Could you check a few things on this model? Use its own coordinates, in mm. A direction names the side the tool comes from. Round coordinates to 2 decimals unless told otherwise and drop trailing zeros. Answer in a Markdown table with one row per item.
Autodesk Fusion 360 part; units mm, degrees
sketch "Sketch1" plane through (0, 0, 0) normal (0, 1, 0) x (1, 0, 0)
  spline S0 degree 3 poles (0, -3.15) (-1.7568, -3.15) (-3.175, -1.7318) (-3.175, 0.025) knots 0 0 0 0 1 1 1 1
  spline S1 degree 3 poles (-3.175, 0.025) (-3.175, 1.7818) (-1.7568, 3.2) (0, 3.2) knots 0 0 0 0 1 1 1 1
  spline S2 degree 3 poles (0, 3.2) (1.7568, 3.2) (3.175, 1.7818) (3.175, 0.025) knots 0 0 0 0 1 1 1 1
  spline S3 degree 3 poles (3.175, 0.025) (3.175, -1.7318) (1.7568, -3.15) (0, -3.15) knots 0 0 0 0 1 1 1 1
  spline S4 degree 3 poles (0, -2.7769) (0.3175, -2.7769) (0.6244, -2.7187) (0.9075, -2.6208) knots 0 0 0 0 1 1 1 1
  line L0 (0.9075, -2.6208) -> (0.0344, -0.7344)
  spline S5 degree 3 poles (0.0344, -0.7344) (0.0238, -0.7238) (0.0238, -0.7) (0, -0.7) knots 0 0 0 0 1 1 1 1
  spline S6 degree 3 poles (0, -0.7) (-0.0238, -0.7) (-0.0238, -0.7238) (-0.0344, -0.7344) knots 0 0 0 0 1 1 1 1
  line L1 (-0.0344, -0.7344) -> (-0.9075, -2.6208)
  line L2 (-1.3494, -2.425) -> (-0.3387, -0.2475)
  spline S7 degree 3 poles (-0.3387, -0.2475) (-0.3175, -0.2025) (-0.2937, -0.1893) (-0.2646, -0.1893) knots 0 0 0 0 1 1 1 1
  line L3 (-0.2646, -0.1893) -> (0.2646, -0.1893)
  spline S8 degree 3 poles (0.2646, -0.1893) (0.2963, -0.1893) (0.3175, -0.2025) (0.3413, -0.2475) knots 0 0 0 0 1 1 1 1
  line L4 (0.3413, -0.2475) -> (1.3388, -2.425)
  spline S9 degree 3 poles (1.3388, -2.425) (1.7568, -2.1869) (2.1167, -1.8456) (2.3707, -1.4381) knots 0 0 0 0 1 1 1 1
  line L5 (2.3707, -1.4381) -> (0.9525, 1.3056)
  spline S10 degree 3 poles (0.9525, 1.3056) (0.9419, 1.3294) (0.926, 1.34) (0.9181, 1.34) knots 0 0 0 0 1 1 1 1
  spline S11 degree 3 poles (0.9181, 1.34) (0.8969, 1.34) (0.8969, 1.3188) (0.8837, 1.3056) knots 0 0 0 0 1 1 1 1
  line L6 (0.8837, 1.3056) -> (0.3413, 0.1044)
  spline S12 degree 3 poles (0.3413, 0.1044) (0.3175, 0.0594) (0.2963, 0.0488) (0.2646, 0.0488) knots 0 0 0 0 1 1 1 1
  line L7 (0.2646, 0.0488) -> (-0.2646, 0.0488)
  spline S13 degree 3 poles (-0.2646, 0.0488) (-0.2937, 0.0488) (-0.3175, 0.0594) (-0.3413, 0.1044) knots 0 0 0 0 1 1 1 1
  line L8 (-0.3413, 0.1044) -> (-0.8837, 1.3056)
  spline S14 degree 3 poles (-0.8837, 1.3056) (-0.8969, 1.3188) (-0.8943, 1.34) (-0.9181, 1.34) knots 0 0 0 0 1 1 1 1
  spline S15 degree 3 poles (-0.9181, 1.34) (-0.9419, 1.34) (-0.9419, 1.3188) (-0.9525, 1.3056) knots 0 0 0 0 1 1 1 1
  line L9 (-0.9525, 1.3056) -> (-2.3812, -1.4381)
  spline S16 degree 3 poles (-2.3812, -1.4381) (-2.1325, -1.8456) (-1.7674, -2.1869) (-1.3494, -2.425) knots 0 0 0 0 1 1 1 1
  line L10 (-2.63, -0.8931) -> (-0.9975, 2.2819)
  spline S17 degree 3 poles (-0.9975, 2.2819) (-0.9763, 2.3269) (-0.9525, 2.3613) (-0.8943, 2.3613) knots 0 0 0 0 1 1 1 1
  spline S18 degree 3 poles (-0.8943, 2.3613) (-0.8387, 2.3613) (-0.8176, 2.3269) (-0.7937, 2.2819) knots 0 0 0 0 1 1 1 1
  line L11 (-0.7937, 2.2819) -> (-0.0344, 0.5912)
  spline S19 degree 3 poles (-0.0344, 0.5912) (-0.0238, 0.57) (-0.0106, 0.5542) (0, 0.5542) knots 0 0 0 0 1 1 1 1
  spline S20 degree 3 poles (0, 0.5542) (0.0238, 0.5542) (0.0238, 0.5806) (0.0344, 0.5912) knots 0 0 0 0 1 1 1 1
  line L12 (0.0344, 0.5912) -> (0.8043, 2.2819)
  spline S21 degree 3 poles (0.8043, 2.2819) (0.8281, 2.3269) (0.8493, 2.3613) (0.9075, 2.3613) knots 0 0 0 0 1 1 1 1
  spline S22 degree 3 poles (0.9075, 2.3613) (0.9631, 2.3613) (0.9869, 2.3269) (1.0081, 2.2819) knots 0 0 0 0 1 1 1 1
  line L13 (1.0081, 2.2819) -> (2.6458, -0.8931)
  spline S23 degree 3 poles (2.6458, -0.8931) (2.7437, -0.61) (2.8019, -0.3031) (2.8019, 0.025) knots 0 0 0 0 1 1 1 1
  spline S24 degree 3 poles (2.8019, 0.025) (2.7887, 1.5569) (1.5319, 2.8269) (0, 2.8269) knots 0 0 0 0 1 1 1 1
  spline S25 degree 3 poles (0, 2.8269) (-1.5319, 2.8269) (-2.7887, 1.5569) (-2.7887, 0.025) knots 0 0 0 0 1 1 1 1
  spline S26 degree 3 poles (-2.7887, 0.025) (-2.7887, -0.2925) (-2.7331, -0.5968) (-2.63, -0.8931) knots 0 0 0 0 1 1 1 1
  arc A0 (-0.9075, -2.6208) -> (0.9075, -2.6208) centre (0, -0.0609) ccw
extrude "Extrude2" add sketch "Sketch1" along normal blind 1
1) I want a section at A-A, the plane z = -0.75. State how many separate pieces and enclosed holes the cut face has, plus the area to 3 significant figures.
Computed:
| item | result |
|---|---|
| separate pieces | 6 |
| enclosed holes | 0 |
| area | 2.95 mm² |
2) Which directions (+Z, -Z, +X, -X, +Y, -Y) give clear straight access to the entire face, cutting with the end or side of a thin tool? Please do faces 1 (the face through (-0.61, 0.49, -0.7)), 2 (the face through (0.66, 0, 1.34)).
Computed:
| item | result |
|---|---|
| face 1 | +Y, -Y |
| face 2 | +Z, -Z, +X, -X, -Y |
3) If we mould it in two halves opening along X, with no side actions, what happens to faces 3 (the face through (-0.45, 0.49, 2.74)), 4 (the face through (0.66, 1, 1.34))? For each: released by +X, released by -X, zero draft, split by the parting line, or undercut.
Computed:
| item | result |
|---|---|
| face 3 | undercut |
| face 4 | zero draft |
4) I need wall thicknesses on line 1 (Z direction, x = 2, y = 0.55); line 2 (X direction, y = 0.15, z = 1); line 3 (Z direction, x = -1.5, y = 0.4). Which ranges of each line are inside material? Lowest first, please.
Computed:
| item | result |
|---|---|
| line 1 | z = -2.49 to -1.97, -0.36 to 0.72, 1.91 to 2.44 |
| line 2 | x = -3.01 to -2.15, -0.69 to -0.16, 0.16 to 0.69, 2.14 to 3.01 |
| line 3 | z = -2.83 to -2.38, -1.3 to -0.25, 2.33 to 2.78 |
